Autodesk Inventor part; units mm, degrees
ref_plane "YZ Plane" through (0, 0, 0) normal (1, 0, 0) x (0, 1, 0)
ref_plane "XZ Plane" through (0, 0, 0) normal (0, 1, 0) x (-1, 0, 0)
ref_plane "XY Plane" through (0, 0, 0) normal (0, 0, 1) x (1, 0, 0)
sketch "스케치1" plane through (0, 0, 0) normal (0, 1, 0) x (-1, 0, 0)
  line L0 (55, 55) -> (-55, 55)
  line L1 (-55, 55) -> (-55, -55)
  line L2 (-55, -55) -> (55, -55)
  line L3 (55, -55) -> (55, 55)
  point P0 (0, 0)
  dimension "d0" = 110
  dimension "d1" = 110
  dimension "d2" = 55
  dimension "d3" = 55
extrude "돌출1" add sketch "스케치1" against normal blind 10
sketch "스케치2" plane through (0, 0, 0) normal (0, 1, 0) x (1, 0, 0)
  circle A0 centre (0, 0) radius 33.5
  circle A1 centre (0, 0) radius 38.5
  circle A2 centre (0, 0) radius 43.5
  line L0 (-55, -55) -> (55, -55)
  line L1 (55, -55) -> (55, 55)
  line L2 (55, 55) -> (-55, 55)
  line L3 (-55, 55) -> (-55, -55)
extrude "돌출2" add sketch "스케치2" along normal blind 2
sketch "스케치3" plane through (0, 0, 0) normal (0, 1, 0) x (1, 0, 0)
  circle A0 centre (0, 0) radius 33.5
  circle A1 centre (-16, 7) radius 3
  circle A2 centre (5, 15) radius 3
  circle A3 centre (16, -7) radius 3
  circle A4 centre (-6, -16) radius 3
  dimension "d8" = 6
  dimension "d9" = 6
  dimension "d10" = 6
  dimension "d11" = 6
extrude "돌출3" cut sketch "스케치3" against normal blind 10 contours A1 | A2 | A3 | A4
fillet "모깎기1" radius 10 4 edges at (-55, -4, -55) (55, -4, -55) (55, -4, 55) (-55, -4, 55)
sketch "스케치5" plane through (0, 2, 0) normal (0, 1, 0) x (1, 0, 0)
  circle A0 centre (0, 0) radius 43.5
  arc A1 (-55, -45) -> (-45, -55) centre (-45, -45) ccw
  line L0 (-45, -55) -> (45, -55)
  arc A2 (45, -55) -> (55, -45) centre (45, -45) ccw
  line L1 (55, -45) -> (55, 45)
  arc A3 (55, 45) -> (45, 55) centre (45, 45) ccw
  line L2 (45, 55) -> (-45, 55)
  arc A4 (-45, 55) -> (-55, 45) centre (-45, 45) ccw
  line L3 (-55, 45) -> (-55, -45)
  circle A5 centre (0, 0) radius 38.5
  circle A6 centre (0, 0) radius 43.5
  circle A7 centre (0, 0) radius 45.5
  dimension "d18" = 91
extrude "돌출5" cut sketch "스케치5" against normal blind 2 contours A7
properties part number "실리콘틀_밑판" material "나일론, 이황화 몰리브덴"
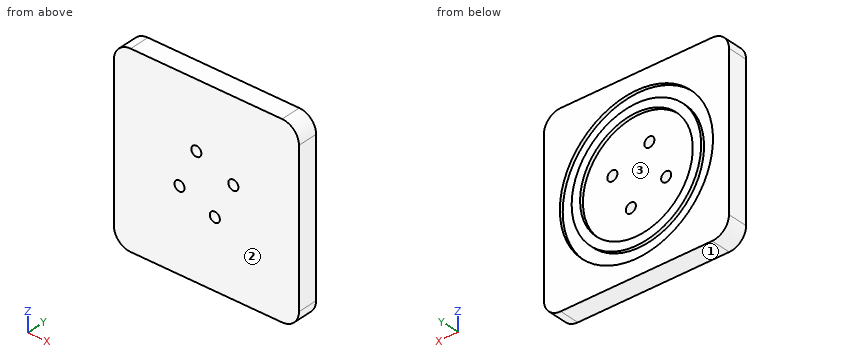
Here's how the part is built. I have some questions about the finished solid (model axes, mm). Face numbers are marked on the shaded views. Round coordinates to 2 decimals unless told otherwise and drop trailing zeros. Loops run counter-clockwise (first coordinate to the right, second up) from the corner with the lowest first, then second, coordinate; pieces in that order, holes last.
1. If we section it at C-C on x = 5: Write out the boundary of the cut face in (y, z).
Answer list:
outline: (-10, -55) - (2, -55) - (2, -45.22) - (0, -45.22) - (0, -38.17) - (2, -38.17) - (2, -33.12) - (0, -33.12) - (0, -18) - (-10, -18) - close; (-10, -12) - (0, -12) - (0, 33.12) - (2, 33.12) - (2, 38.17) - (0, 38.17) - (0, 45.22) - (2, 45.22) - (2, 55) - (-10, 55) - close
2. If we section it at B-B on z = 16: Write out the boundary of the cut face in (x, y).
Answer list:
outline: (-55, -10) - (-9, -10) - (-9, 0) - (-29.43, 0) - (-29.43, 2) - (-35.02, 2) - (-35.02, 0) - (-42.59, 0) - (-42.59, 2) - (-55, 2) - close; (-3, -10) - (55, -10) - (55, 2) - (42.59, 2) - (42.59, 0) - (35.02, 0) - (35.02, 2) - (29.43, 2) - (29.43, 0) - (-3, 0) - close
3. We'd pull the mould along Z, two halves only. Please class the marked faces 1, 2 and 3: +Z half, -Z half, draft (parallel to the pull), parting line (faces both ways), or undercut.
Answer list:
face 1: -Z half
face 2: draft
face 3: undercut
4. If I drill on line 1 along Z through (x, y) = (0, 0.45); line 2 along Z through (x, y) = (-6, -5); line 3 along Z through (x, y) = (-16, -4.75), over which ranges is the centre line in solid material (lowest first)?
Answer list:
line 1: z = -55 to -45.5, -38.5 to -33.5, 33.5 to 38.5, 45.5 to 55
line 2: z = -55 to 13, 19 to 55
line 3: z = -55 to -10, -4 to 55
5. For P1, Ø5.5, axis at x = -6, z = 16, coming from the +Y side; P2, Ø9.5, axis at x = 5, z = -15, coming from the +Y side, each with a flat end and sliding along its axis, tell me the tip position at first contact or that it passes through.
Answer list:
P1: passes through
P2: stops at y = 0
6. If we section it at D-D on z = 0: Write out the boundary of the cut face in (x, y), plus the area to 3 significant figures.
Answer list:
outline: (-55, -10) - (55, -10) - (55, 2) - (45.5, 2) - (45.5, 0) - (38.5, 0) - (38.5, 2) - (33.5, 2) - (33.5, 0) - (-33.5, 0) - (-33.5, 2) - (-38.5, 2) - (-38.5, 0) - (-45.5, 0) - (-45.5, 2) - (-55, 2) - close
area: 1,160 mm2
7. If we section it at A-A on y = -1.5: Write out the boundary of the cut face in (x, z), plus the area to 3 significant figures.
Answer list:
outline: (-55, -45) arc R10 ccw to (-45, -55) - (45, -55) arc R10 ccw to (55, -45) - (55, 45) arc R10 ccw to (45, 55) - (-45, 55) arc R10 ccw to (-55, 45) - close; hole circle Ø6 at (-16, -7); hole circle Ø6 at (-6, 16); hole circle Ø6 at (5, -15); hole circle Ø6 at (16, 7)
area: 11,900 mm2
